Study the drawing (mm; zero at the part's minimum x, y, z) and answer. A direction names the side the tool comes from. Round coordinates to 2 decimals unless told otherwise and drop trailing zeros. Order: outer loops, then holes, each group sorted by start corner. A loop starts at its lowest first (then second) coordinate and runs counter-clockwise, first axis right, second up. Notation, with made-up numbers: (46, 48.5) - (76, 48.5) arc R13 cw to (76, 52.5) - close; hole circle Ø6 at (25, -25.75). An arc over 180 degrees is marked (long way). Use one line per item in the form item = value. Start each with the question number.
Q1. Given P1, Ø5, axis at x = 8.5, y = 20, coming from the +Z side; P2, Ø2, axis at y = 5.5, z = 2.5, coming from the +X side; P3, Ø3, axis at x = 4.5, z = 4.5, coming from the -Y side, each flat-ended and moving along its own axis, determine where each tip first touches the part or whether it passes through.
Q2. Which of the six approach directions +Z, -Z, +X, -X, +Y, -Y give full straight-line access (tool end or side, diameter ignored) to the marked faces 4, 5 and 6?
Q3. For a pull along Z with two mould halves and no side action, classify the marked faces 1, 2 and 3 as +Z half, -Z half, draft (parallel to the pull), parting line (faces both ways), or undercut.
Q4. The part is cut by section A-A on y = 6. Determine the outline of the cut face in (x, z) (1 decimal).
Q5. Find the intervals of material crossed by line 1 (Y direction, x = 9.75, z = 7.5) (1 decimal); line 2 (Y direction, x = 5.75, z = 6.75); line 3 (Z direction, x = 5.5, y = 2) (1 decimal), in increasing order. Write a range as [from, to].
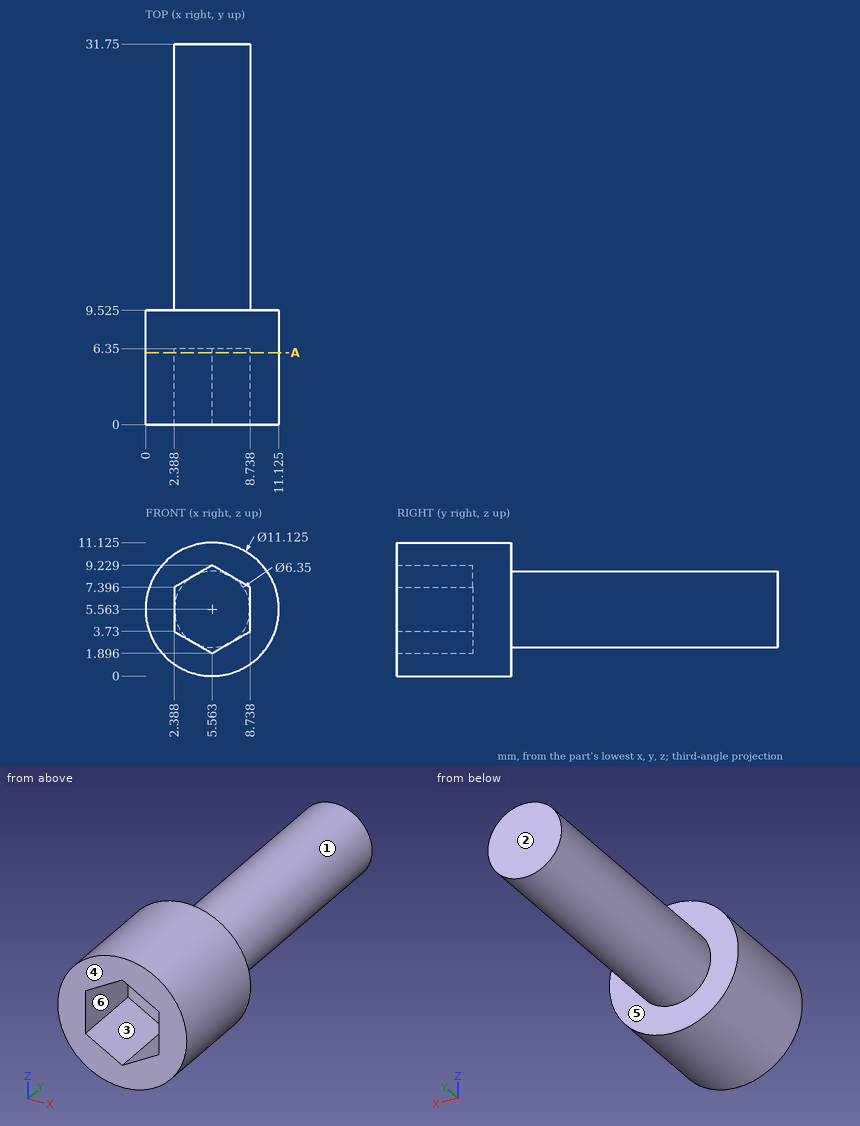
Found:
q1.P1 = 8.71
q1.P2 = 10.73
q1.P3 = 6.35
q2.face_4 = +Z, -Z, +X, -X, -Y
q2.face_5 = +Y
q2.face_6 = -Y
q3.face_1 = parting line
q3.face_2 = draft
q3.face_3 = undercut
q4.outline = circle Ø11.1 at (5.6, 5.6); hole (2.4, 3.7) - (5.6, 1.9) - (8.7, 3.7) - (8.7, 7.4) - (5.6, 9.2) - (2.4, 7.4) - close
q5.line_1 = [0, 9.5]
q5.line_2 = [6.35, 31.75]
q5.line_3 = [0, 1.9], [9.2, 11.1]
